from build123d import *

# Parameters (mm, degrees)
SKETCH1_R                       = 19.05
BOSS_EXTRUDE1_DEPTH             = 263.525
SKETCH2_W                       = 258.7625
SKETCH2_H                       = 12.7
CUT_EXTRUDE1_DEPTH              = 265.898528922
CUT_EXTRUDE1_DEPTH_BACK         = 265.898528922
SKETCH8_W                       = 25.4
SKETCH8_H                       = 0.79375
F_1_1_DIAMETER_HOLE2_D          = 6.35
F_16_0_177_DIAMETER_HOLE1_D     = 4.4958
F_16_0_177_DIAMETER_HOLE1_DEPTH = 25.4
F_16_0_177_DIAMETER_HOLE1_TIP   = 1.350674586
BOSS_EXTRUDE2_START             = 1.5875
SKETCH15_R                      = 8.89
SKETCH15_R_2                    = 6.35
BOSS_EXTRUDE2_DEPTH             = 1.5875


with BuildPart() as part:
    # Sketch1 → Boss-Extrude1 (new body)
    with BuildSketch(Plane(origin=(0, 0, 0), x_dir=(0, 0, -1), z_dir=(1, 0, 0))):
        Circle(SKETCH1_R)
    extrude(amount=BOSS_EXTRUDE1_DEPTH)

    # Sketch2 → Cut-Revolve1 (revolve, cut)
    with BuildSketch(Plane.XY, mode=Mode.PRIVATE) as cut_revolve1_sk:
        with Locations((129.38125, 12.7)):
            Rectangle(SKETCH2_W, SKETCH2_H)
    revolve(cut_revolve1_sk.sketch.rotate(Axis((-16.52066387, 0, 0), (1, 0, 0)), 90), axis=Axis((-16.52066387, 0, 0), (1, 0, 0)), mode=Mode.SUBTRACT)

    # Sketch8 → Cut-Extrude1 (cut, two sides: drawn at the far end of the back side and taken through both)
    with BuildSketch(Plane(origin=(0, 0, 0), x_dir=(1, 0, 0), z_dir=(0, 1, 0)).offset(-CUT_EXTRUDE1_DEPTH_BACK)):
        with Locations((12.7, 5.953125)):
            Rectangle(SKETCH8_W, SKETCH8_H)
        with Locations((12.7, -5.953125)):
            Rectangle(SKETCH8_W, SKETCH8_H)
    extrude(amount=CUT_EXTRUDE1_DEPTH + CUT_EXTRUDE1_DEPTH_BACK, mode=Mode.SUBTRACT)

    # 1 (1) Diameter Hole2 (through all)
    with Locations(Plane(origin=(0, 0, -5.55625), x_dir=(-1, 0, 0), z_dir=(0, 0, -1))):
        with Locations((-6.35, 0)):
            Hole(F_1_1_DIAMETER_HOLE2_D / 2)

    # #16 (0.177) Diameter Hole1
    with Locations(Plane.ZY.offset(-258.7625)):
        with Locations((9.525, 9.525), (-9.525, -9.525), (-9.525, 9.525), (9.525, -9.525)):
            Hole(F_16_0_177_DIAMETER_HOLE1_D / 2, depth=F_16_0_177_DIAMETER_HOLE1_DEPTH)
            with Locations((0, 0, -(F_16_0_177_DIAMETER_HOLE1_DEPTH + F_16_0_177_DIAMETER_HOLE1_TIP / 2))):  # 118° drill point
                Cone(0, F_16_0_177_DIAMETER_HOLE1_D / 2, F_16_0_177_DIAMETER_HOLE1_TIP, mode=Mode.SUBTRACT)

    # Sketch15 → Boss-Extrude2 (add)
    with BuildSketch(Plane(origin=(263.525, 0, 0), x_dir=(0, 0, -1), z_dir=(1, 0, 0)).offset(BOSS_EXTRUDE2_START)):
        Circle(SKETCH15_R)
        with Locations(Location((0, 0, 0), (0, 0, 180))):
            Circle(SKETCH15_R_2, mode=Mode.SUBTRACT)
    extrude(amount=-BOSS_EXTRUDE2_DEPTH)


solid = part.part
Design review of the part built by this model. Coordinates are the model's own, in mm. A direction names the side the tool comes from. Give positions to 0.01 mm unless a question says otherwise; leave off trailing zeros. Write each loop counter-clockwise with the first axis right and the second up, starting at its lowest first coordinate (ties: lowest second). Pieces come first, ordered by that corner, then holes. Notation, with made-up numbers: M -15.5,56.5 L 25.5,56.5 A18 ccw 25.5,88.5 Z; hole C 16.5,-12.75 d4. An arc over 180 degrees is marked long. Answer as a JSON object with one key per item and string values. Group by question number.
1) For line 1 along Y through (x, z) = (264.3, 0); line 2 along X through (y, z) = (1.5, 16.5) (1 decimal); line 3 along Z through (x, y) = (14.5, 1.5), list the stretches that pass through material, from the lowest coordinate up.
2) We need section C-C (x = 164.5). Give the boundary of the cut face in (y, z), and give its area (3 significant figures).
3) Mouldability with a two-part tool opening along Y and no side actions: class faces 5 (the face through (261.18, 9.62, 11.77)), 6 (the face through (131.193, -0.279, -6.344)), 7 (the face through (0, 0, 0)), 8 (the face through (261.18, -8.85, -11.67)) as released by +Y, released by -Y, zero draft, split by the parting line, or undercut.
4) Clearance check with flat-ended pins moving along their axes: pin 1 Ø7 at (x, y) = (17, 0.5) entering from +Z; pin 2 Ø4 at (y, z) = (9.525, 9.525) entering from +X; pin 3 Ø7 at (y, z) = (-9.525, 9.525) entering from +X (3 decimals); pin 4 Ø5 at (x, z) = (177, -6.5) entering from +Y. State where each tip first meets the part, or that it passes through.
5) We need section D-D (z = 15). Give the boundary of the cut face in (x, y) (1 decimal).
6) Tool access review of faces 1 (the face through (258.762, -5, 5)), 2 (the face through (263.525, 0, 0)), 3 (the face through (16, 0, 5.556)), 4 (the face through (16, 0, -5.556)): name each direction out of +Z, -Z, +X, -X, +Y, -Y from which nothing blocks a thin tool from reaching the whole face with its end or side.
Answer key:
{
 "1": {"line 1": "y = -8.89 to -6.35, 6.35 to 8.89", "line 2": "x = 258.8 to 263.5", "line 3": "z = -5.56 to 5.56"},
 "2": {"outline": "C 0,0 d12.7", "area": "127 mm²"},
 "3": {"face 5": "undercut", "face 6": "split by the parting line", "face 7": "zero draft", "face 8": "undercut"},
 "4": {"pin 1": "stops at z = 5.56", "pin 2": "passes through", "pin 3": "stops at x = 263.525", "pin 4": "stops at y = 4.93"},
 "5": {"outline": "M 258.8,-11.7 L 263.5,-11.7 L 263.5,11.7 L 258.8,11.7 Z"},
 "6": {"face 1": "-X", "face 2": "+X", "face 3": "+Z, -X, +Y, -Y", "face 4": "-Z, -X, +Y, -Y"}
}
